Autodesk Inventor part; units mm, degrees
ref_plane "YZ Plane" through (0, 0, 0) normal (1, 0, 0) x (0, 1, 0)
ref_plane "XZ Plane" through (0, 0, 0) normal (0, 1, 0) x (-1, 0, 0)
ref_plane "XY Plane" through (0, 0, 0) normal (0, 0, 1) x (1, 0, 0)
sketch "Sketch1" plane through (0, 0, 0) normal (0, 1, 0) x (-1, 0, 0)
  line L0 (20, 45) -> (-20, 45)
  line L1 (-20, 45) -> (-20, -45)
  line L2 (-20, -45) -> (20, -45)
  line L3 (20, -45) -> (20, 45)
  line L4 (20, 45) -> (-20, -45) construction
  line L5 (-20, 45) -> (20, -45) construction
  arc A0 (-20, -45) -> (20, -45) centre (0, -45) ccw
  line L6 (20, -45) -> (30, -45)
  line L7 (30, -45) -> (30, 45)
  line L8 (30, 45) -> (20, 45)
  line L9 (20, 45) -> (20, -45)
  point P0 (0, 0)
  dimension "d0" = 40
  dimension "d1" = 90
  dimension "d7" = 10
  dimension "d8" = 90
extrude "Extrusion1" add sketch "Sketch1" along normal blind 3.6
sketch "Sketch2" plane through (0, 3.6, 0) normal (0, 1, 0) x (1, 0, 0)
  arc A0 (20, 45) -> (-20, 45) centre (0, 45) ccw
  circle A1 centre (0, 45) radius 5.15
  point P0 (0, 0)
  dimension "d4" = 10.3
extrude "Extrusion2" cut sketch "Sketch2" against normal blind 3.6
fillet "Fillet1" radius 4 3 edges at (-20, 1.8, -45) (-30, 1.8, -45) (20, 1.8, 45)
sketch "Sketch3" plane through (0, 0, 0) normal (0, -1, 0) x (1, 0, 0)
  circle A0 centre (-5, 20) radius 22.5
  line L0 (20, 41) -> (20, -45)
  line L1 (-30, 45) -> (16, 45)
  point P0 (0, 0)
  point P1 (-26, 45)
  dimension "d10" = 45
  dimension "d11" = 25
  dimension "d12" = 25
extrude "Extrusion3" cut sketch "Sketch3" against normal blind 10
sketch "Sketch4" plane through (0, 0, 0) normal (0, -1, 0) x (1, 0, 0)
  circle A0 centre (15.5, 40.5) radius 1.625
  circle A1 centre (-25.5, -40.5) radius 1.625
  circle A2 centre (15.5, -19.5) radius 1.625
  line L0 (-30, -41) -> (-30, 45)
  line L1 (-23.6643, -45) -> (-26, -45)
  line L2 (20, 41) -> (20, -45)
  line L3 (-30, 45) -> (16, 45)
  point P0 (0, 0)
  point P1 (-30, 41)
  point P2 (-26, 45)
  dimension "d15" = 3.25
  dimension "d17" = 3.25
  dimension "d18" = 3.25
  dimension "d19" = 4.5
  dimension "d20" = 4.5
  dimension "d21" = 4.5
  dimension "d23" = 4.5
  dimension "d24" = 4.5
  dimension "d27" = 60
extrude "Extrusion4" cut sketch "Sketch4" against normal blind 10
fillet "Fillet2" radius 25 1 edges at (-30, 1.8, 45)
properties part number "p1"
Work out the finished part from the listing and answer in its coordinate system (mm). A direction names the side the tool comes from. Coordinates: 2 decimals unless noted, no trailing zeros. Loops run counter-clockwise (first coordinate to the right, second up) from the corner with the lowest first, then second, coordinate; pieces in that order, holes last.
1) Section D-D (z = 23.5) is taken. Give the vertices of the cut face in (x, y).
Results:
outline: (-29.75, 0) - (-27.23, 0) - (-27.23, 3.6) - (-29.75, 3.6) - close; (17.23, 0) - (20, 0) - (20, 3.6) - (17.23, 3.6) - close
2) Consider probe 1 along Z at (x, y) = (0, 1.1); probe 2 along X at (y, z) = (2.65, 40); probe 3 along Z at (x, y) = (15.5, 1.5) (3 decimals). Determine where each line is inside the solid, lowest interval first.
Results:
probe 1: z = -65 to -50.15, -39.85 to -1.94, 41.94 to 45
probe 2: x = -20 to -15.31, 5.31 to 13.95, 17.05 to 20
probe 3: z = -57.639 to -21.125, -17.875 to 10.726, 29.274 to 38.875, 42.125 to 45
3) Flat-ended cylindrical pins translate along their axes: pin 1 (2 mm diameter, centred on y = 2, z = -53.5, fed in from -X); pin 2 (1.2 mm diameter, centred on x = -24.5, y = 2, fed in from -Z); pin 3 (2.5 mm diameter, centred on x = 15.5, z = 40.5, fed in from -Y). Find the tip coordinate at first contact, or state that the pin passes through.
Results:
pin 1: stops at x = -18.54
pin 2: stops at z = -45
pin 3: passes through
4) For a pull along Z with two mould halves and no side action, classify faces 1 (the cylindrical face through (-28.797, 1.825, -43.859)), 2 (the flat face through (-30, 2, -11)), 3 (the cylindrical face through (16.25, 1.77, 39.06)) as +Z half, -Z half, draft (parallel to the pull), parting line (faces both ways), or undercut.
Results:
face 1: -Z half
face 2: draft
face 3: undercut
5) For faces 4 (the cylindrical face through (-22.871, 1.825, 37.482)), 5 (the flat face through (-25, 2, -45)), determine the directions among +Z, -Z, +X, -X, +Y, -Y from which every point of the face is accessible in a straight line to the end or side of a thin tool.
Results:
face 4: +Z, -X, +Y, -Y
face 5: -Z, -X, +Y, -Y
6) Section C-C (x = -1) is taken. Give the vertices of the cut face in (y, z), plus the area to 3 significant figures.
Results:
outline: (0, -64.97) - (3.6, -64.97) - (3.6, -50.05) - (0, -50.05) - close; (0, -39.95) - (3.6, -39.95) - (3.6, -2.14) - (0, -2.14) - close; (0, 42.14) - (3.6, 42.14) - (3.6, 45) - (0, 45) - close
area: 200 mm2
7) Section B-B (x = -7) is taken. Give the vertices of the cut face in (y, z) (3 decimals), plus the area to 3 significant figures.
Results:
outline: (0, -63.735) - (3.6, -63.735) - (3.6, -2.411) - (0, -2.411) - close; (0, 42.411) - (3.6, 42.411) - (3.6, 44.92) - (0, 44.92) - close
area: 230 mm2
8) Section A-A (y = 2.2) is taken. Give the vertices of the cut face in (x, z) (3 decimals), plus the area to 3 significant figures.
Results:
outline: (-30, -41) arc R4 ccw to (-26, -45) - (-23.664, -45) arc R4 cw to (-19.72, -48.333) arc R20 ccw to (20, -45) - (20, 41) arc R4 ccw to (16, 45) - (-5, 45) arc R25 ccw to (-30, 20) - close; hole circle Ø45 at (-5, 20); hole circle Ø3.25 at (-25.5, -40.5); hole circle Ø10.3 at (0, -45); hole circle Ø3.25 at (15.5, -19.5); hole circle Ø3.25 at (15.5, 40.5)
area: 3,290 mm2
